Geometry check sheet. Reference: the model listing, model coordinates, mm. A direction names the side the tool comes from. Coordinates: 2 decimals unless noted, no trailing zeros. Write each loop counter-clockwise with the first axis right and the second up, starting at its lowest first coordinate (ties: lowest second). Pieces come first, ordered by that corner, then holes. Notation, with made-up numbers: (38.5, 46.5) -> (56.5, 46.5) arc R14 cw to (56.5, 73.5) -> close; hole circle Ø8 at (7, 28.5). An arc over 180 degrees is marked (long way). Answer as CSV lines item,"result".
```python
from build123d import *

# Parameters (mm, degrees)
F0_R     = 15
F1_DEPTH = 6
F2_R     = 10.5
F3_DEPTH = 3
F5_D     = 6.8
F5_DEPTH = 10


with BuildPart() as f1:
    # F0 (on Front) → F1 (new body)
    with BuildSketch(Plane.XZ):
        Circle(F0_R)
    extrude(amount=F1_DEPTH)

    # F2 (on face) → F3 (join)
    with BuildSketch(Plane.XZ.offset(6)):
        Circle(F2_R)
    extrude(amount=F3_DEPTH)

    # F5
    with Locations(Plane.XZ.offset(9)):
        with Locations((0, 0)):
            Hole(F5_D / 2, depth=F5_DEPTH)


solid = f1.part
```
Item 1: Cross-section at D-D, the plane z = 8.5. Record the cut outline in (x, y), plus the area to 3 significant figures.
Responses:
outline,"(-12.36, -6) -> (-6.16, -6) -> (-6.16, -9) -> (6.16, -9) -> (6.16, -6) -> (12.36, -6) -> (12.36, 0) -> (-12.36, 0) -> close"
area,"185 mm2"
Item 2: Cross-section at B-B, the plane z = 0. Record the cut outline in (x, y), plus the area to 3 significant figures.
Responses:
outline,"(-15, -6) -> (-10.5, -6) -> (-10.5, -9) -> (-3.4, -9) -> (-3.4, 0) -> (-15, 0) -> close; (3.4, -9) -> (10.5, -9) -> (10.5, -6) -> (15, -6) -> (15, 0) -> (3.4, 0) -> close"
area,"182 mm2"
Item 3: Thickness scan on probe 1 along Z at (x, y) = (0, -2.5); probe 2 along Z at (x, y) = (0, -7); probe 3 along Y at (x, z) = (-7.75, 10). Record the ranges inside material, lowest first.
Responses:
probe 1,"z = -15 to -3.4, 3.4 to 15"
probe 2,"z = -10.5 to -3.4, 3.4 to 10.5"
probe 3,"y = -6 to 0"
Item 4: Cross-section at A-A, the plane x = 0. Record the cut outline in (y, z).
Responses:
outline,"(-9, -10.5) -> (-6, -10.5) -> (-6, -15) -> (0, -15) -> (0, -3.4) -> (-9, -3.4) -> close; (-9, 3.4) -> (0, 3.4) -> (0, 15) -> (-6, 15) -> (-6, 10.5) -> (-9, 10.5) -> close"
Item 5: Depth check by flat-ended pin: pin 1 Ø4 at (x, z) = (0, 0) entering from -Y; pin 2 Ø4 at (y, z) = (-3, -11.5) entering from -X; pin 3 Ø3 at (x, y) = (-10.5, -8) entering from +Z; pin 4 Ø4 at (x, y) = (3, -7.5) entering from +Z. Enter the tip coordinate at first touch or a pass-through.
Responses:
pin 1,"passes through"
pin 2,"stops at x = -11.61"
pin 3,"stops at z = 5.41"
pin 4,"stops at z = 14.91"
Item 6: Cross-section at C-C, the plane y = -7.5. Record the cut outline in (x, z), plus the area to 3 significant figures.
Responses:
outline,"circle Ø21 at (0, 0); hole circle Ø6.8 at (0, 0)"
area,"310 mm2"
Item 7: Set-up check for faces 1 (the flat face through (3.1, -6, 10.2)), 2 (the cylindrical face through (-14.985, -2.958, 0.66)): record each of +Z, -Z, +X, -X, +Y, -Y from which the full face is reachable in a straight line by a thin tool's end or side.
Responses:
face 1,"-Y"
face 2,"+Y, -Y"
Item 8: Release check for a two-part mould opening along Z. For faces 3 (the cylindrical face through (0.74, -4.44, -3.32)), 4 (the cylindrical face through (10, -7.5, 3.2)), 5 (the flat face through (5, -9, 0)) record: +Z half, -Z half, draft (parallel to the pull), parting line (faces both ways), or undercut.
Responses:
face 3,"undercut"
face 4,"parting line"
face 5,"draft"
